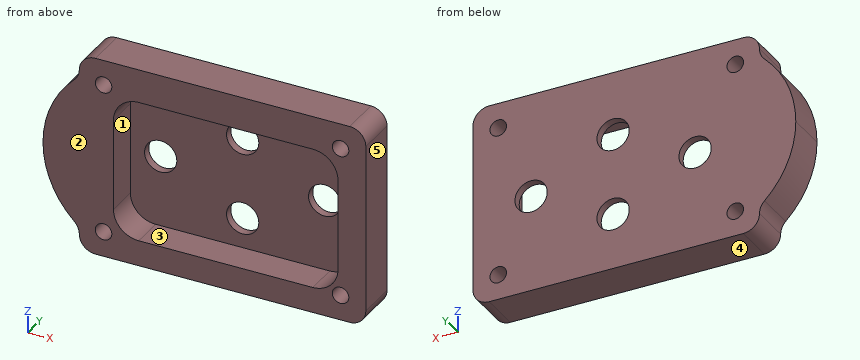
```python
from build123d import *

# Parameters (mm, degrees)
SKETCH1_W           = 40
SKETCH1_H           = 25
BOSS_EXTRUDE1_DEPTH = 5
CUT_EXTRUDE1_DEPTH  = 25.109126902
SKETCH4_W           = 8
SKETCH4_H           = 25
BOSS_EXTRUDE2_DEPTH = 5
FILLET1_R           = 2
SKETCH5_R           = 1.025
CUT_EXTRUDE2_DEPTH  = 25.109126902
SKETCH6_R           = 2
CUT_EXTRUDE3_DEPTH  = 25.109126902
CUT_EXTRUDE4_DEPTH  = 4


with BuildPart() as part:
    # Sketch1 → Boss-Extrude1 (new body)
    with BuildSketch(Plane(origin=(0, 0, 0), x_dir=(1, 0, 0), z_dir=(0, 1, 0))):
        Rectangle(SKETCH1_W, SKETCH1_H)
    extrude(amount=BOSS_EXTRUDE1_DEPTH)

    # Sketch2 → Cut-Extrude1 (cut, through all)
    with BuildSketch(Plane(origin=(0, 5, 0), x_dir=(1, 0, 0), z_dir=(0, 1, 0))):
        with BuildLine():
            ThreePointArc((-20, 0), (-16.338834759, 8.83883477), (-7.499999984, 12.5))
            Line((-7.499999984, 12.5), (-20, 12.5))
            Line((-20, 12.5), (-20, 0))
        make_face()
        with BuildLine():
            Line((-20, -12.5), (-7.50000001, -12.5))
            ThreePointArc((-7.50000001, -12.5), (-16.338834768, -8.838834761), (-20, 0))
            Line((-20, 0), (-20, -12.5))
        make_face()
    extrude(amount=-CUT_EXTRUDE1_DEPTH, mode=Mode.SUBTRACT)

    # Sketch4 → Boss-Extrude2 (add, through all)
    with BuildSketch(Plane(origin=(0, 5, 0), x_dir=(1, 0, 0), z_dir=(0, 1, 0))):
        with Locations((-11.5, 0)):
            Rectangle(SKETCH4_W, SKETCH4_H)
    extrude(amount=-BOSS_EXTRUDE2_DEPTH)

    # Fillet1
    fillet1_edges = [part.edges().sort_by_distance(p)[0] for p in [
        (20, 2.5, 12.5),
        (20, 2.5, -12.5),
        (-15.5, 2.5, -12.5),
        (-15.5, 2.5, 12.5),
        (-15.5, 2.5, 9.604686356),
        (-15.5, 2.5, -9.604686356),
    ]]
    fillet(fillet1_edges, radius=FILLET1_R - 0.0001)  # a hair under: the kernel refuses the full size

    # Sketch5 → Cut-Extrude2 (cut, through all)
    with BuildSketch(Plane(origin=(0, 5, 0), x_dir=(1, 0, 0), z_dir=(0, 1, 0))):
        with Locations(Location((-12.496001599, 9.37, 0), (0, 0, 270))):
            Circle(SKETCH5_R)
        with Locations(Location((-12.496001599, -9.37, 0), (0, 0, 270))):
            Circle(SKETCH5_R)
        with Locations(Location((16.87, 9.37, 0), (0, 0, 270))):
            Circle(SKETCH5_R)
        with Locations(Location((16.87, -9.37, 0), (0, 0, 270))):
            Circle(SKETCH5_R)
    extrude(amount=-CUT_EXTRUDE2_DEPTH, mode=Mode.SUBTRACT)

    # Sketch6 → Cut-Extrude3 (cut, through all)
    with BuildSketch(Plane.XZ):
        with Locations(Location((-7.519296648, -0.485, 0), (0, 0, 270))):
            Circle(SKETCH6_R)
        with Locations(Location((2.640703352, 4.595, 0), (0, 0, 270))):
            Circle(SKETCH6_R)
        with Locations(Location((12.800703352, -0.485, 0), (0, 0, 270))):
            Circle(SKETCH6_R)
        with Locations(Location((2.640703352, -5.565, 0), (0, 0, 270))):
            Circle(SKETCH6_R)
    extrude(amount=-CUT_EXTRUDE3_DEPTH, mode=Mode.SUBTRACT)

    # Sketch7 → Cut-Extrude4 (cut)
    with BuildSketch(Plane.XZ):
        with BuildLine():
            Line((-11.269296648, -6.19), (-11.269296648, 5.22))
            ThreePointArc((-11.269296648, 5.22), (-10.354005339, 7.429708691), (-8.144296648, 8.345))
            Line((-8.144296648, 8.345), (13.425703352, 8.345))
            ThreePointArc((13.425703352, 8.345), (15.635412043, 7.429708691), (16.550703352, 5.22))
            Line((16.550703352, 5.22), (16.550703352, -6.19))
            ThreePointArc((16.550703352, -6.19), (15.635412043, -8.399708691), (13.425703352, -9.315))
            Line((13.425703352, -9.315), (-8.144296648, -9.315))
            ThreePointArc((-8.144296648, -9.315), (-10.354005339, -8.399708691), (-11.269296648, -6.19))
        make_face()
    extrude(amount=-CUT_EXTRUDE4_DEPTH, mode=Mode.SUBTRACT)


solid = part.part
```
Part model, mm, in its own coordinate system. Face numbers are marked on the shaded views. A direction names the side the tool comes from. Round coordinates to 2 decimals unless told otherwise and drop trailing zeros. Loops run counter-clockwise (first coordinate to the right, second up) from the corner with the lowest first, then second, coordinate; pieces in that order, holes last. Notation, with made-up numbers: (23, 49.25) -> (65, 49.25) arc R26 cw to (65, 74.25) -> close; hole circle Ø8 at (81, -17.75). An arc over 180 degrees is marked (long way). Use CSV: the item, a comma, the result in double quotes. Start each with the question number.
1) Wall check: L1, parallel to Z at x = 13, y = 3.1 (3 decimals); L2, parallel to X at y = 3.9, z = -9.5; L3, parallel to X at y = 3.5, z = 9.37 (3 decimals). Give the ranges that are in metal, low to high. Write a range as [from, to].
2) Cut at D-D, the plane x = 4. Write the cut outline in (y, z) (3 decimals).
3) Cut at B-B, the plane z = 3.75. Write the cut outline in (x, y), plus the area to 3 significant figures.
4) Cut at C-C, the plane y = 2.2. Give the number of separate pieces and of enclosed holes in the cut face, plus the area to 3 significant figures.
5) Which spindle directions (+Z, -Z, +X, -X, +Y, -Y) get a long thin tool onto all of the face, cutting with end or side? Do the marked faces 1 and 2. Say none if no direction does.
6) Cut at A-A, the plane x = -1.5. Write the cut outline in (y, z) (3 decimals), plus the area to 3 significant figures.
7) Pull direction Z, two halves, no side cores. Call the marked faces 3, 4 and 5: +Z half, -Z half, draft (parallel to the pull), parting line (faces both ways), or undercut.
8) Drop flat-ended pins along their axis: P1, Ø3, axis at x = 2.64, z = -5.56, coming from the -Y side; P2, Ø9, axis at x = 0, z = -4, coming from the -Y side. Give the stop position or say it passes through.
Determined:
1,L1,"z = [-12.5, -9.315], [8.345, 12.5]"
1,L2,"x = [-15.77, -13.51], [-11.48, 15.85], [17.89, 20]"
1,L3,"x = [-15.85, -13.521], [-11.471, 15.845], [17.895, 20]"
2,outline,"(0, -12.5) -> (5, -12.5) -> (5, -7.032) -> (4, -7.032) -> (4, -9.315) -> (0, -9.315) -> close; (0, 8.345) -> (4, 8.345) -> (4, 6.062) -> (5, 6.062) -> (5, 12.5) -> (0, 12.5) -> close; (4, -4.098) -> (5, -4.098) -> (5, 3.128) -> (4, 3.128) -> close"
3,outline,"(-19.42, 0) -> (-11.27, 0) -> (-11.27, 4) -> (0.83, 4) -> (0.83, 5) -> (-19.42, 5) -> close; (4.45, 4) -> (16.55, 4) -> (16.55, 0) -> (20, 0) -> (20, 5) -> (4.45, 5) -> close"
3,area,"82.2 mm2"
4,separate pieces,"1"
4,enclosed holes,"5"
4,area,"448 mm2"
5,face 1,"-Y"
5,face 2,"+Z, -Z, +X, -X, -Y"
6,outline,"(0, -12.5) -> (5, -12.5) -> (5, 12.5) -> (0, 12.5) -> (0, 8.345) -> (4, 8.345) -> (4, -9.315) -> (0, -9.315) -> close"
6,area,"54.4 mm2"
7,face 3,"undercut"
7,face 4,"-Z half"
7,face 5,"draft"
8,P1,"passes through"
8,P2,"stops at y = 4"
